Geometry: see drawing. Coordinates: mm, zero at the bounding-box minimum. A direction names the side the tool comes from. Coordinates: 2 decimals unless noted, no trailing zeros. Order: outer loops, then holes, each group sorted by start corner. A loop starts at its lowest first (then second) coordinate and runs counter-clockwise, first axis right, second up.
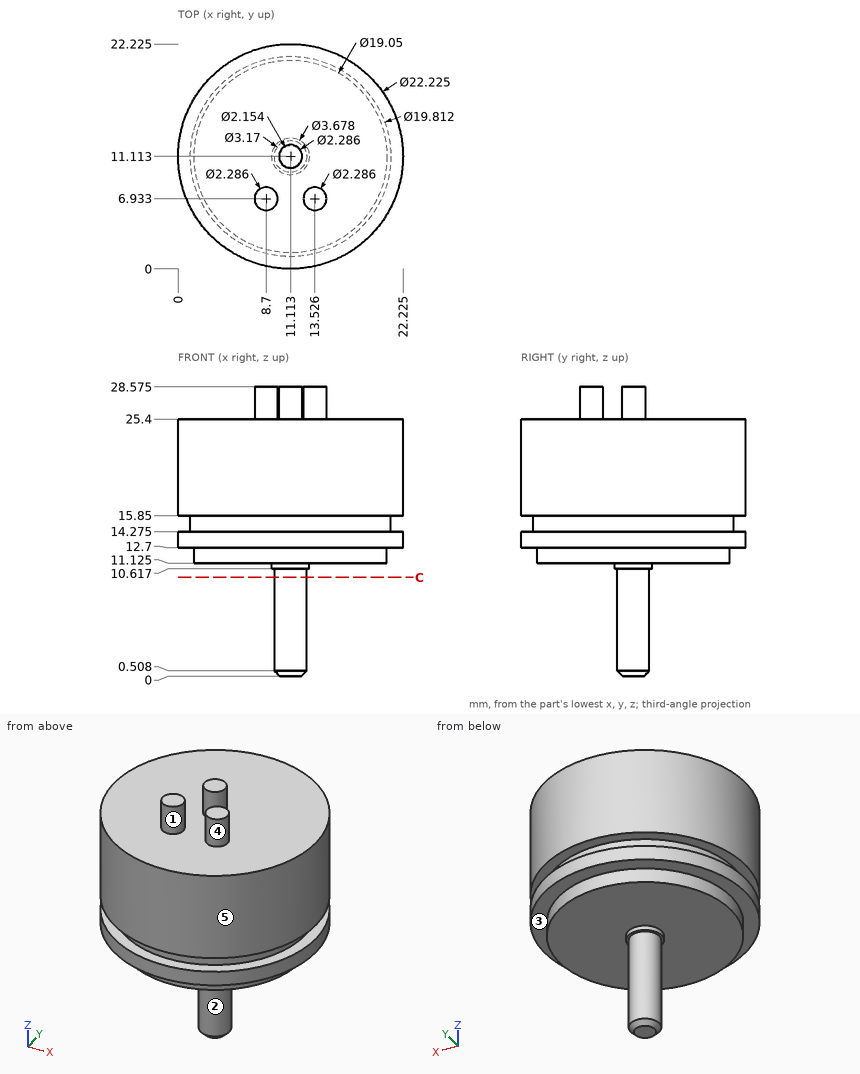
Q1. Section query C-C on z = 9.75. Output: boundary loops of the cut face in (x, y) (1 decimal).
Solutions:
outline: circle Ø3.2 at (11.1, 11.1)
Q2. Pin query (flat end, axial travel): P1, Ø1.5, axis at x = 5, y = 4, coming from the -Z side (1 decimal); P2, Ø1.5, axis at y = 2.5, z = 19.5, coming from the +X side (1 decimal); P3, Ø10, axis at y = 2.5, z = 17, coming from the -X side. Return the tip coordinate at first contact, or that it passes through.
Solutions:
P1: stops at z = 11.1
P2: stops at x = 19
P3: stops at x = 0.6
Q3. Pull-direction query (X, two-part tool) for the marked faces 1, 2 and 3; classes: pulls with the +X half, pulls with the -X half, needs draft (parallel to the pull), parting line crosses it, or undercut.
Solutions:
face 1: undercut
face 2: parting line crosses it
face 3: needs draft
Q4. Material intervals for line 1 along Z through (x, y) = (11, 16) (1 decimal); line 2 along X through (y, z) = (11.5, 23); line 3 along Y through (x, z) = (15, 18.75), sorted ascending.
Solutions:
line 1: z = 11.1 to 25.4
line 2: x = 0.01 to 22.22
line 3: y = 0.7 to 21.52
Q5. Set-up query: the marked faces 4 and 5. Return all of +Z, -Z, +X, -X, +Y, -Y with unobstructed straight access to the full face (end or side cutting, diameter ignored); none if empty.
Solutions:
face 4: +Z
face 5: +Z, -Z
